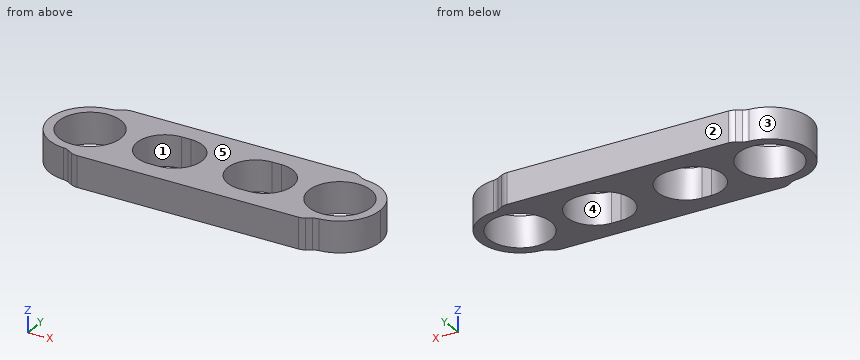
from build123d import *

# Parameters (mm, degrees)
SKETCH_1_R          = 3.5
EXTRUDE_1_DEPTH     = 5
CUT_EXTRUDE_2_DEPTH = 49.347699015
SKETCH_6_R          = 5
CUT_EXTRUDE_3_DEPTH = 6
CUT_EXTRUDE_4_DEPTH = 10
FILLET_1_R          = 2


with BuildPart() as part:
    # 草图1 → 凸台-拉伸1 (new body)
    with BuildSketch(Plane.XY):
        with BuildLine():
            Line((0, 7.5), (40, 7.5))
            ThreePointArc((40, 7.5), (47.5, 0), (40, -7.5))
            Line((40, -7.5), (0, -7.5))
            ThreePointArc((0, -7.5), (-7.5, 0), (0, 7.5))
        make_face()
        Circle(SKETCH_1_R, mode=Mode.SUBTRACT)
        with Locations((40, 0)):
            Circle(SKETCH_1_R, mode=Mode.SUBTRACT)
    extrude(amount=EXTRUDE_1_DEPTH)

    # 草图3 → 切除-拉伸2 (cut, through all)
    with BuildSketch(Plane.XY.offset(5)):
        with BuildLine():
            ThreePointArc((0, -6.5), (-6.5, 0), (0, 6.5))
            Line((0, 6.5), (1.732050808, 7.5))
            Line((1.732050808, 7.5), (0, 7.5))
            ThreePointArc((0, 7.5), (-7.5, 0), (0, -7.5))
            Line((0, -7.5), (1.732050808, -7.5))
            Line((1.732050808, -7.5), (0, -6.5))
        make_face()
        with BuildLine():
            Line((40, 7.5), (38.267949192, 7.5))
            Line((38.267949192, 7.5), (40, 6.5))
            ThreePointArc((40, 6.5), (44.596194078, 4.596194078), (46.5, 0))
            ThreePointArc((46.5, 0), (44.596194078, -4.596194078), (40, -6.5))
            Line((40, -6.5), (38.267949192, -7.5))
            Line((38.267949192, -7.5), (40, -7.5))
            ThreePointArc((40, -7.5), (47.5, 0), (40, 7.5))
        make_face()
    extrude(amount=-CUT_EXTRUDE_2_DEPTH, mode=Mode.SUBTRACT)

    # 草图6 → 切除-拉伸3 (cut)
    with BuildSketch(Plane.XY.offset(5)):
        Circle(SKETCH_6_R)
        with Locations((40, 0)):
            Circle(SKETCH_6_R)
    extrude(amount=-CUT_EXTRUDE_3_DEPTH, mode=Mode.SUBTRACT)

    # 草图4 → 切除-拉伸4 (cut)
    with BuildSketch(Plane.XY.offset(5)):
        with BuildLine():
            Line((12, 4.5), (13.5, 4.5))
            ThreePointArc((13.5, 4.5), (18, 0), (13.5, -4.5))
            Line((13.5, -4.5), (12, -4.5))
            ThreePointArc((12, -4.5), (7.5, 0), (12, 4.5))
        make_face()
        with BuildLine():
            Line((28, 4.5), (26.5, 4.5))
            ThreePointArc((26.5, 4.5), (22, 0), (26.5, -4.5))
            Line((26.5, -4.5), (28, -4.5))
            ThreePointArc((28, -4.5), (32.5, 0), (28, 4.5))
        make_face()
    extrude(amount=-CUT_EXTRUDE_4_DEPTH, mode=Mode.SUBTRACT)

    # 圆角1
    fillet_1_edges = [part.edges().sort_by_distance(p)[0] for p in [
        (0, 6.5, 2.5),
        (0, -6.5, 2.5),
        (1.732050808, -7.5, 2.5),
        (1.732050808, 7.5, 2.5),
        (40, 6.5, 2.5),
        (38.267949192, 7.5, 2.5),
        (38.267949192, -7.5, 2.5),
        (40, -6.5, 2.5),
    ]]
    fillet(fillet_1_edges, radius=FILLET_1_R)


solid = part.part
The model under review builds one solid part; all positions refer to its coordinate system, in mm. Face numbers are marked on the shaded views. A direction names the side the tool comes from. Round coordinates to 2 decimals unless told otherwise and drop trailing zeros. Order: outer loops, then holes, each group sorted by start corner. A loop starts at its lowest first (then second) coordinate and runs counter-clockwise, first axis right, second up. Notation, with made-up numbers: (48.5, -2) - (97.5, -2) arc R21 cw to (97.5, 14) - close; hole circle Ø11 at (-16.75, -18.5). An arc over 180 degrees is marked (long way). Use one line per item in the form item = value.
Q1. Clearance check with flat-ended pins moving along their axes: P1, Ø1, axis at x = -0.5, z = 4, coming from the +Y side; P2, Ø1.5, axis at y = -4, z = 1.5, coming from the -X side; P3, Ø6, axis at x = 0, y = 0, coming from the +Z side. State where each tip first meets the part, or that it passes through.
Response values:
P1 = 6.56
P2 = -5.63
P3 = through
Q2. To check wall thickness, follow line 1 (X direction, y = -3.5, z = 2.4); line 2 (Y direction, x = 28, z = 0.9); line 3 (Y direction, x = 0, z = 2.75). State the ranges of each line that lie inside material, in increasing order.
Response values:
line_1 = -5.48 to -3.57, 3.57 to 9.17, 16.33 to 23.67, 30.83 to 36.43, 43.57 to 45.48
line_2 = -7.5 to -4.5, 4.5 to 7.5
line_3 = -6.56 to -5, 5 to 6.56
Q3. Mouldability with a two-part tool opening along X and no side actions: class the marked faces 1, 2 and 3 as pulls with the +X half, pulls with the -X half, needs draft (parallel to the pull), parting line crosses it, or undercut.
Response values:
face_1 = undercut
face_2 = needs draft
face_3 = pulls with the -X half
Q4. Add section D-D on y = 2.25. Give the boundary of the cut face in (x, z), then the cut area to 3 significant figures.
Response values:
outline = (-6.1, 0) - (-4.47, 0) - (-4.47, 5) - (-6.1, 5) - close; (4.47, 0) - (8.1, 0) - (8.1, 5) - (4.47, 5) - close; (17.4, 0) - (22.6, 0) - (22.6, 5) - (17.4, 5) - close; (31.9, 0) - (35.53, 0) - (35.53, 5) - (31.9, 5) - close; (44.47, 0) - (46.1, 0) - (46.1, 5) - (44.47, 5) - close
area = 78.7 mm^2
Q5. Add section B-B on z = 4.25. Give the boundary of the cut face in (x, y), then the cut area to 3 significant figures.
Response values:
outline = (-0.44, -6.49) arc R2 cw to (0.43, -6.75) - (1.27, -7.23) arc R2 ccw to (2.27, -7.5) - (37.73, -7.5) arc R2 ccw to (38.73, -7.23) - (39.57, -6.75) arc R2 cw to (40.44, -6.49) arc R6.5 ccw to (40.44, 6.49) arc R2 cw to (39.57, 6.75) - (38.73, 7.23) arc R2 ccw to (37.73, 7.5) - (2.27, 7.5) arc R2 ccw to (1.27, 7.23) - (0.43, 6.75) arc R2 cw to (-0.44, 6.49) arc R6.5 ccw to start; hole circle Ø10 at (0, 0); hole (12, -4.5) - (13.5, -4.5) arc R4.5 ccw to (13.5, 4.5) - (12, 4.5) arc R4.5 ccw to start; hole (26.5, -4.5) - (28, -4.5) arc R4.5 ccw to (28, 4.5) - (26.5, 4.5) arc R4.5 ccw to start; hole circle Ø10 at (40, 0)
area = 418 mm^2
Q6. Add section A-A on y = -0.75. Give the boundary of the cut face in (x, z).
Response values:
outline = (-6.46, 0) - (-4.94, 0) - (-4.94, 5) - (-6.46, 5) - close; (4.94, 0) - (7.56, 0) - (7.56, 5) - (4.94, 5) - close; (17.94, 0) - (22.06, 0) - (22.06, 5) - (17.94, 5) - close; (32.44, 0) - (35.06, 0) - (35.06, 5) - (32.44, 5) - close; (44.94, 0) - (46.46, 0) - (46.46, 5) - (44.94, 5) - close
Q7. Tool access review of the marked faces 4 and 5: name each direction out of +Z, -Z, +X, -X, +Y, -Y from which nothing blocks a thin tool from reaching the whole face with its end or side.
Response values:
face_4 = +Z, -Z
face_5 = +Z, +X, -X, +Y, -Y
Q8. Add section C-C on x = 31. Give the boundary of the cut face in (y, z), then the cut area to 3 significant figures.
Response values:
outline = (-7.5, 0) - (-3.35, 0) - (-3.35, 5) - (-7.5, 5) - close; (3.35, 0) - (7.5, 0) - (7.5, 5) - (3.35, 5) - close
area = 41.5 mm^2
